```python
from build123d import *

# Parameters (mm, degrees)
SKETCH2_R           = 52.5
SKETCH2_R_2         = 47.5
BOSS_EXTRUDE1_DEPTH = 25
SKETCH2_6_R         = 47.5
SKETCH2_6_R_2       = 45
BOSS_EXTRUDE5_DEPTH = 19
SKETCH2_7_R         = 45
SKETCH2_7_R_2       = 26.5
BOSS_EXTRUDE6_DEPTH = 10


with BuildPart() as part:
    # Sketch2 → Boss-Extrude1 (new body)
    with BuildSketch(Plane.XY):
        Circle(SKETCH2_R)
        Circle(SKETCH2_R_2, mode=Mode.SUBTRACT)
    extrude(amount=BOSS_EXTRUDE1_DEPTH)

    # Sketch2<6> → Boss-Extrude5 (add)
    with BuildSketch(Plane.XY):
        Circle(SKETCH2_6_R)
        Circle(SKETCH2_6_R_2, mode=Mode.SUBTRACT)
    extrude(amount=BOSS_EXTRUDE5_DEPTH)

    # Sketch2<7> → Boss-Extrude6 (add)
    with BuildSketch(Plane.XY):
        Circle(SKETCH2_7_R)
        Circle(SKETCH2_7_R_2, mode=Mode.SUBTRACT)
    extrude(amount=BOSS_EXTRUDE6_DEPTH)


solid = part.part
```
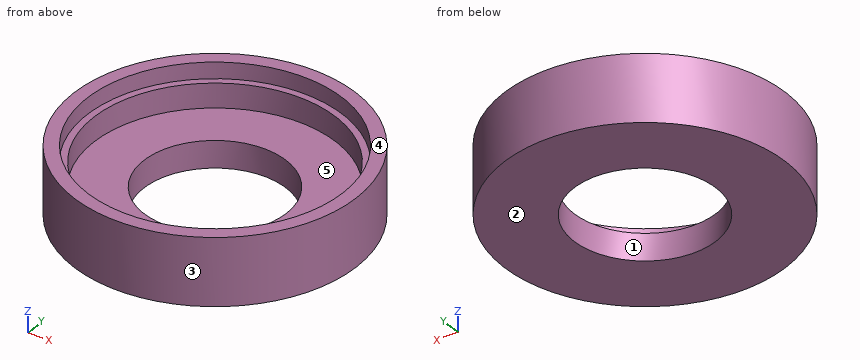
Check sheet for the modelled part. Datum: model origin and axes. Units: mm. Face numbers are marked on the shaded views. A direction names the side the tool comes from. Coordinates: 2 decimals unless noted, no trailing zeros. Order: outer loops, then holes, each group sorted by start corner. A loop starts at its lowest first (then second) coordinate and runs counter-clockwise, first axis right, second up. Notation, with made-up numbers: M 68.25,41 L 92.25,41 A19 cw 92.25,47 Z; hole C -11,86 d5. An arc over 180 degrees is marked long. Write each question's results on one line, items separated by ' | '. Start each with the question number.
1. Mould release check, pull along Y, two halves, no side actions. Record for the marked faces 1, 2 and 3: +Y half, -Y half, draft (parallel to the pull), parting line (faces both ways), or undercut.
2. Cross-section at D-D on z = 4.5. Record the cut outline in (x, y).
3. Access from +Z, -Z, +X, -X, +Y, -Y to the whole of each face (thin tool, end or side, straight path). Record for the marked faces 4 and 5.
4. Cross-section at A-A on x = 0. Record the cut outline in (y, z).
5. Cross-section at C-C on x = 31. Record the cut outline in (y, z).
6. Go/stop test with flat-tipped pins: P1, Ø12, axis at y = -22.5, z = 6.5, coming from the -X side; P2, Ø8, axis at y = 35.5, z = 20, coming from the +X side; P3, Ø3, axis at y = 30.5, z = 15.5, coming from the -X side; P4, Ø4, axis at x = -42, y = -37, coming from the -Z side. Record where each tip stops, or that it passes through.
7. Material ranges on probe 1 along Y at (x, z) = (0, 12); probe 2 along Y at (x, z) = (0, 22.55), recorded low to high.
Checks:
1) face 1: undercut | face 2: draft | face 3: parting line
2) outline: C 0,0 d105; hole C 0,0 d53
3) face 4: +Z, +X, -X, +Y, -Y | face 5: +Z
4) outline: M -52.5,0 L -26.5,0 L -26.5,10 L -45,10 L -45,19 L -47.5,19 L -47.5,25 L -52.5,25 Z; M 26.5,0 L 52.5,0 L 52.5,25 L 47.5,25 L 47.5,19 L 45,19 L 45,10 L 26.5,10 Z
5) outline: M -42.37,0 L 42.37,0 L 42.37,25 L 35.99,25 L 35.99,19 L 32.62,19 L 32.62,10 L -32.62,10 L -32.62,19 L -35.99,19 L -35.99,25 L -42.37,25 Z
6) P1: stops at x = -49.84 | P2: stops at x = 42 | P3: stops at x = -43.76 | P4: passes through
7) probe 1: y = -52.5 to -45, 45 to 52.5 | probe 2: y = -52.5 to -47.5, 47.5 to 52.5
